Design review of the part built by this model. Coordinates are the model's own, in mm. Face numbers are marked on the shaded views. A direction names the side the tool comes from. Coordinates: 2 decimals unless noted, no trailing zeros. Order: outer loops, then holes, each group sorted by start corner. A loop starts at its lowest first (then second) coordinate and runs counter-clockwise, first axis right, second up. Notation, with made-up numbers: M 72,-34.5 L 105,-34.5 A17 cw 105,-8.5 Z; hole C -28,54 d11. An arc over 180 degrees is marked long. Answer as a JSON object with one key per item and string values.
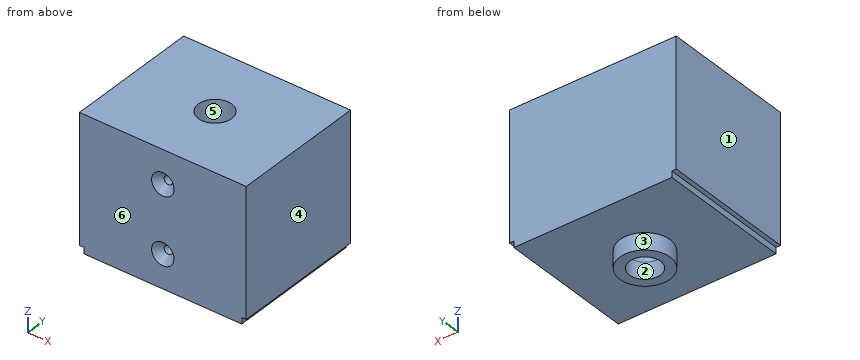
from build123d import *

# Parameters (mm, degrees)
F1_DEPTH        = 40
F2_R            = 7.5
F3_DEPTH        = 5
F10_D           = 2.5
F10_DEPTH       = 16
F10_CSINK_D     = 6.72
F10_CSINK_ANGLE = 90
F10_TIP         = 0.7510757738


with BuildPart() as f1:
    # F0 (on Front) → F1 (new body)
    with BuildSketch(Plane.XZ):
        Polygon((24.9, 40), (-24.9, 40), (-24.9, 1.85), (-23.575, 1.85), (-23.575, 0), (23.575, 0), (23.575, 1.85), (24.9, 1.85), align=None)
    extrude(amount=F1_DEPTH)

    # F2 (on face) → F3 (join)
    with BuildSketch(Plane(origin=(0, 0, 0), x_dir=(1, 0, 0), z_dir=(0, 0, -1))):
        with Locations((0, 20)):
            Circle(F2_R)
    extrude(amount=F3_DEPTH)


with BuildPart() as f7:
    # F6 (on line) → F7 (revolve)
    with BuildSketch(Plane(origin=(0, -20, 0), x_dir=(-1, 0, 0), z_dir=(0, 1, 0))):
        Polygon((4.8, 0), (4.95, 40), (0, 40), (0, 0), (0, -5), (4.65, -5), (4.715, 0), align=None)
    revolve(axis=Axis((0, -20, 30.4776426257), (0, 0, 1)))


with BuildPart() as f1_1:
    add(f1.part)

    # F8: cut F7
    add(f7.part, mode=Mode.SUBTRACT)

    # F10
    with Locations(Plane.XZ.offset(40)):
        with Locations((0, 30), (0, 10)):
            CounterSinkHole(F10_D / 2, F10_CSINK_D / 2, depth=F10_DEPTH, counter_sink_angle=F10_CSINK_ANGLE)
            with Locations((0, 0, -(F10_DEPTH + F10_TIP / 2))):  # 118° drill point
                Cone(0, F10_D / 2, F10_TIP, mode=Mode.SUBTRACT)


solid = f1_1.part
1) Insertion check: pin 1 Ø4 at (x, z) = (0, 10) entering from -Y; pin 2 Ø1 at (x, y) = (-13, -31.5) entering from -Z; pin 3 Ø0.6 at (y, z) = (-19.5, 1.5) entering from +X (3 decimals). Each pin has a flat end and moves straight along its axis. Give the tip position at first contact, or say it passes through.
Taken from the geometry:
{"pin 1": "stops at y = -38.64", "pin 2": "stops at z = 0", "pin 3": "stops at x = 23.575"}
2) Add section D-D (z = 24.5). State the section outline as (x, y) points, and give its area (3 significant figures).
Taken from the geometry:
{"outline": "M -24.9,-40 L 24.9,-40 L 24.9,0 L -24.9,0 Z; hole C 0,-20 d9.78", "area": "1,920 mm2"}
3) Tool access review of the marked faces 1, 2 and 3: name each direction out of +Z, -Z, +X, -X, +Y, -Y from which nothing blocks a thin tool from reaching the whole face with its end or side.
Taken from the geometry:
{"face 1": "+Z, -Z, -X, +Y, -Y", "face 2": "+Z", "face 3": "-Z"}
4) To check wall thickness, follow L1, parallel to Z at x = 0, y = -29.5; L2, parallel to X at y = -30, z = 30; L3, parallel to Z at x = 13, y = -10. State the ranges of each line that lie inside material, in increasing order.
Taken from the geometry:
{"L1": "z = 0 to 8.75, 11.25 to 28.75, 31.25 to 40", "L2": "x = -24.9 to -1.25, 1.25 to 24.9", "L3": "z = 0 to 40"}
5) Add section A-A (y = -29). State the section outline as (x, z) points (3 decimals).
Taken from the geometry:
{"outline": "M -24.9,1.85 L -23.575,1.85 L -23.575,0 L 23.575,0 L 23.575,1.85 L 24.9,1.85 L 24.9,40 L -24.9,40 Z; hole C 0,10 d2.5; hole C 0,30 d2.5"}
6) Mouldability with a two-part tool opening along X and no side actions: class the marked faces 4, 5 and 6 as released by +X, released by -X, zero draft, split by the parting line, or undercut.
Taken from the geometry:
{"face 4": "released by +X", "face 5": "undercut", "face 6": "zero draft"}
7) Add section B-B (y = -5.5). State the section outline as (x, z) points (3 decimals).
Taken from the geometry:
{"outline": "M -24.9,1.85 L -23.575,1.85 L -23.575,0 L 23.575,0 L 23.575,1.85 L 24.9,1.85 L 24.9,40 L -24.9,40 Z"}
